Input: part model. Units: mm. Frame: model coordinates. Face numbers are marked on the shaded views. A direction names the side the tool comes from. Coordinates: 2 decimals unless noted, no trailing zeros. Order: outer loops, then holes, each group sorted by start corner. A loop starts at its lowest first (then second) coordinate and runs counter-clockwise, first axis right, second up. Notation, with made-up numbers: (-31, -15) -> (14, -15) arc R23 cw to (14, 21) -> close; hole circle Ø8 at (23.5, -22). An arc over 180 degrees is marked (long way). Use one line per item in the form item = value. Start each with the question number.
1) Section query C-C on y = 15. Output: boundary loops of the cut face in (x, z) (3 decimals).
2) Draft query along X for the marked faces 1, 2, 3 and 4. Return one class per face: pulls with the +X half, pulls with the -X half, needs draft (parallel to the pull), parting line crosses it, or undercut.
3) Section query D-D on y = -16. Output: boundary loops of the cut face in (x, z).
4) Pin query (flat end, axial travel): pin 1 (6 mm diameter, centred on y = -22, z = -9, fed in from -X); pin 2 (9 mm diameter, centred on x = 76.5, z = -70, fed in from +Y); pin 3 (0.9 mm diameter, centred on x = -32.5, y = -1.5, fed in from +Z); pin 4 (25 mm diameter, centred on x = 85.5, y = -15.5, fed in from +Z). Return the tip coordinate at first contact, or that it passes through.
5) Ray query, line 1 along Z through (x, y) = (76.5, 12.75) (3 decimals); line 2 along Z through (x, y) = (76.5, -0.75) (3 decimals); line 3 along Y through (x, z) = (-15, -1.5). Return the intervals inside material, ascending.
6) Access query for the marked faces 5, 6, 7 and 8. Directions: +Z, -Z, +X, -X, +Y, -Y. A direction counts if a zero-diameter tool reaches every point of the face in a straight line with its end or side. Return the directions, or none.
from build123d import *

# Parameters (mm, degrees)
F1_DEPTH       = 25
F2_DEPTH       = 10
F3_DEPTH       = 30
F4_DEPTH       = 20
F5_DEPTH       = 8
F6_SIZE2       = 5
F6_SIZE        = 5
F8_D           = 14.75
F8_CBORE_D     = 22.25
F8_CBORE_DEPTH = 14
F9_R           = 7.49999


# Not quite as in the source:
# - a fillet or chamfer is up to 0.001 mm smaller than in the source, because OpenCascade refuses the exact size


with BuildPart() as f1:
    # F0 (on Front) → F1 (new body)
    with BuildSketch(Plane.XZ):
        with BuildLine():
            Line((106.5, -40), (106.5, 55))
            Line((106.5, 55), (48.7497216032, 55))
            ThreePointArc((48.7497216032, 55), (42.4942891815, 52.8018949761), (38.9888762464, 47.1739130435))
            ThreePointArc((38.9888762464, 47.1739130435), (10.7462120246, -4.2462120246), (-40.6739130435, -32.4888762464))
            ThreePointArc((-40.6739130435, -32.4888762464), (-46.3018949761, -35.9942891815), (-48.5, -42.2497216032))
            Line((-48.5, -42.2497216032), (-48.5, -100))
            Line((-48.5, -100), (46.5, -100))
            Line((46.5, -100), (46.5, -55))
            ThreePointArc((46.5, -55), (50.8933982822, -44.3933982822), (61.5, -40))
            Line((61.5, -40), (106.5, -40))
        make_face()
        with BuildLine():
            ThreePointArc((-29.5, -91), (-36.5710678119, -88.0710678119), (-39.5, -81))
            Line((-39.5, -81), (-39.5, -49.2476414861))
            ThreePointArc((-39.5, -49.2476414861), (-37.481834214, -43.2234965193), (-32.2419354839, -39.630896205))
            ThreePointArc((-32.2419354839, -39.630896205), (17.1101730553, -10.6101730553), (46.130896205, 38.7419354839))
            ThreePointArc((46.130896205, 38.7419354839), (49.7234965193, 43.981834214), (55.7476414861, 46))
            Line((55.7476414861, 46), (87.5, 46))
            ThreePointArc((87.5, 46), (94.5710678119, 43.0710678119), (97.5, 36))
            Line((97.5, 36), (97.5, -21))
            ThreePointArc((97.5, -21), (94.5710678119, -28.0710678119), (87.5, -31))
            Line((87.5, -31), (61.5, -31))
            ThreePointArc((61.5, -31), (44.5294372515, -38.0294372515), (37.5, -55))
            Line((37.5, -55), (37.5, -81))
            ThreePointArc((37.5, -81), (34.5710678119, -88.0710678119), (27.5, -91))
            Line((27.5, -91), (-29.5, -91))
        make_face(mode=Mode.SUBTRACT)
        with BuildLine():
            Line((96.5, 100), (-96.5, 100))
            ThreePointArc((-96.5, 100), (-103.5710678119, 97.0710678119), (-106.5, 90))
            Line((-106.5, 90), (-106.5, -90))
            ThreePointArc((-106.5, -90), (-103.5710678119, -97.0710678119), (-96.5, -100))
            Line((-96.5, -100), (-63.5, -100))
            Line((-63.5, -100), (-63.5, -42.2497216032))
            ThreePointArc((-63.5, -42.2497216032), (-58.0047374401, -26.6111405489), (-43.9347826087, -17.8476082112))
            ThreePointArc((-43.9347826087, -17.8476082112), (0.1396103068, 6.3603896932), (24.3476082112, 50.4347826087))
            ThreePointArc((24.3476082112, 50.4347826087), (33.1111405489, 64.5047374401), (48.7497216032, 70))
            Line((48.7497216032, 70), (106.5, 70))
            Line((106.5, 70), (106.5, 90))
            ThreePointArc((106.5, 90), (103.5710678119, 97.0710678119), (96.5, 100))
        make_face()
        with BuildLine():
            ThreePointArc((14.7304288624, 91), (-11.3221396288, 8.044605666), (-97.5, -3.5187051029))
            Line((-97.5, -3.5187051029), (-97.5, 91))
            Line((-97.5, 91), (14.7304288624, 91))
        make_face(mode=Mode.SUBTRACT)
        with BuildLine():
            Line((-97.5, 91), (-97.5, -3.5187051029))
            ThreePointArc((-97.5, -3.5187051029), (-11.3221396288, 8.044605666), (14.7304288624, 91))
            Line((14.7304288624, 91), (-97.5, 91))
        make_face()
        with BuildLine():
            Line((-39.5, -49.2476414861), (-39.5, -81))
            ThreePointArc((-39.5, -81), (-36.5710678119, -88.0710678119), (-29.5, -91))
            Line((-29.5, -91), (27.5, -91))
            ThreePointArc((27.5, -91), (34.5710678119, -88.0710678119), (37.5, -81))
            Line((37.5, -81), (37.5, -55))
            ThreePointArc((37.5, -55), (44.5294372515, -38.0294372515), (61.5, -31))
            Line((61.5, -31), (87.5, -31))
            ThreePointArc((87.5, -31), (94.5710678119, -28.0710678119), (97.5, -21))
            Line((97.5, -21), (97.5, 36))
            ThreePointArc((97.5, 36), (94.5710678119, 43.0710678119), (87.5, 46))
            Line((87.5, 46), (55.7476414861, 46))
            ThreePointArc((55.7476414861, 46), (49.7234965193, 43.981834214), (46.130896205, 38.7419354839))
            ThreePointArc((46.130896205, 38.7419354839), (17.1101730553, -10.6101730553), (-32.2419354839, -39.630896205))
            ThreePointArc((-32.2419354839, -39.630896205), (-37.481834214, -43.2234965193), (-39.5, -49.2476414861))
        make_face()
        with BuildLine():
            Line((106.5, 55), (106.5, 70))
            Line((106.5, 70), (48.7497216032, 70))
            ThreePointArc((48.7497216032, 70), (33.1111405489, 64.5047374401), (24.3476082112, 50.4347826087))
            ThreePointArc((24.3476082112, 50.4347826087), (0.1396103068, 6.3603896932), (-43.9347826087, -17.8476082112))
            ThreePointArc((-43.9347826087, -17.8476082112), (-58.0047374401, -26.6111405489), (-63.5, -42.2497216032))
            Line((-63.5, -42.2497216032), (-63.5, -100))
            Line((-63.5, -100), (-48.5, -100))
            Line((-48.5, -100), (-48.5, -42.2497216032))
            ThreePointArc((-48.5, -42.2497216032), (-46.3018949761, -35.9942891815), (-40.6739130435, -32.4888762464))
            ThreePointArc((-40.6739130435, -32.4888762464), (10.7462120246, -4.2462120246), (38.9888762464, 47.1739130435))
            ThreePointArc((38.9888762464, 47.1739130435), (42.4942891815, 52.8018949761), (48.7497216032, 55))
            Line((48.7497216032, 55), (106.5, 55))
        make_face()
        with BuildLine():
            Line((106.5, -90), (106.5, -40))
            Line((106.5, -40), (61.5, -40))
            ThreePointArc((61.5, -40), (50.8933982822, -44.3933982822), (46.5, -55))
            Line((46.5, -55), (46.5, -100))
            Line((46.5, -100), (96.5, -100))
            ThreePointArc((96.5, -100), (103.5710678119, -97.0710678119), (106.5, -90))
        make_face()
    extrude(amount=-F1_DEPTH)

    # F0 (on Front) → F2 (join)
    with BuildSketch(Plane.XZ):
        with BuildLine():
            Line((106.5, -90), (106.5, -40))
            Line((106.5, -40), (61.5, -40))
            ThreePointArc((61.5, -40), (50.8933982822, -44.3933982822), (46.5, -55))
            Line((46.5, -55), (46.5, -100))
            Line((46.5, -100), (96.5, -100))
            ThreePointArc((96.5, -100), (103.5710678119, -97.0710678119), (106.5, -90))
        make_face()
    extrude(amount=F2_DEPTH)

    # F0 (on Front) → F3 (join)
    with BuildSketch(Plane.XZ):
        with BuildLine():
            Line((106.5, 55), (106.5, 70))
            Line((106.5, 70), (48.7497216032, 70))
            ThreePointArc((48.7497216032, 70), (33.1111405489, 64.5047374401), (24.3476082112, 50.4347826087))
            ThreePointArc((24.3476082112, 50.4347826087), (0.1396103068, 6.3603896932), (-43.9347826087, -17.8476082112))
            ThreePointArc((-43.9347826087, -17.8476082112), (-58.0047374401, -26.6111405489), (-63.5, -42.2497216032))
            Line((-63.5, -42.2497216032), (-63.5, -100))
            Line((-63.5, -100), (-48.5, -100))
            Line((-48.5, -100), (-48.5, -42.2497216032))
            ThreePointArc((-48.5, -42.2497216032), (-46.3018949761, -35.9942891815), (-40.6739130435, -32.4888762464))
            ThreePointArc((-40.6739130435, -32.4888762464), (10.7462120246, -4.2462120246), (38.9888762464, 47.1739130435))
            ThreePointArc((38.9888762464, 47.1739130435), (42.4942891815, 52.8018949761), (48.7497216032, 55))
            Line((48.7497216032, 55), (106.5, 55))
        make_face()
    extrude(amount=F3_DEPTH)

    # F0 (on Front) → F4 (cut)
    with BuildSketch(Plane.XZ):
        with BuildLine():
            Line((-39.5, -49.2476414861), (-39.5, -81))
            ThreePointArc((-39.5, -81), (-36.5710678119, -88.0710678119), (-29.5, -91))
            Line((-29.5, -91), (27.5, -91))
            ThreePointArc((27.5, -91), (34.5710678119, -88.0710678119), (37.5, -81))
            Line((37.5, -81), (37.5, -55))
            ThreePointArc((37.5, -55), (44.5294372515, -38.0294372515), (61.5, -31))
            Line((61.5, -31), (87.5, -31))
            ThreePointArc((87.5, -31), (94.5710678119, -28.0710678119), (97.5, -21))
            Line((97.5, -21), (97.5, 36))
            ThreePointArc((97.5, 36), (94.5710678119, 43.0710678119), (87.5, 46))
            Line((87.5, 46), (55.7476414861, 46))
            ThreePointArc((55.7476414861, 46), (49.7234965193, 43.981834214), (46.130896205, 38.7419354839))
            ThreePointArc((46.130896205, 38.7419354839), (17.1101730553, -10.6101730553), (-32.2419354839, -39.630896205))
            ThreePointArc((-32.2419354839, -39.630896205), (-37.481834214, -43.2234965193), (-39.5, -49.2476414861))
        make_face()
    extrude(amount=-F4_DEPTH, mode=Mode.SUBTRACT)

    # F0 (on Front) → F5 (join)
    with BuildSketch(Plane.XZ):
        with BuildLine():
            Line((-97.5, 91), (-97.5, -3.5187051029))
            ThreePointArc((-97.5, -3.5187051029), (-11.3221396288, 8.044605666), (14.7304288624, 91))
            Line((14.7304288624, 91), (-97.5, 91))
        make_face()
    extrude(amount=F5_DEPTH)

    # F6
    f6_edges = [f1.edges().sort_by_distance(p)[0] for p in [
        (-41.384786, -8, 91),
        (-97.5, -8, 43.740647),
        (-11.32214, -8, 8.044606),
    ]]
    chamfer(f6_edges, length=F6_SIZE, length2=F6_SIZE2)

    # F8 (through all)
    with Locations(Plane.XZ.offset(10)):
        with Locations((76.5, -70)):
            CounterBoreHole(F8_D / 2, F8_CBORE_D / 2, F8_CBORE_DEPTH)

    # F9 (radius 7.5 in the source; OpenCascade refuses exactly that, so slightly less here)
    f9_edges = [f1.edges().sort_by_distance(p)[0] for p in [
        (-48.5, -30, -71.124861),
        (-63.5, -30, -71.124861),
    ]]
    fillet(f9_edges, radius=F9_R)


solid = f1.part
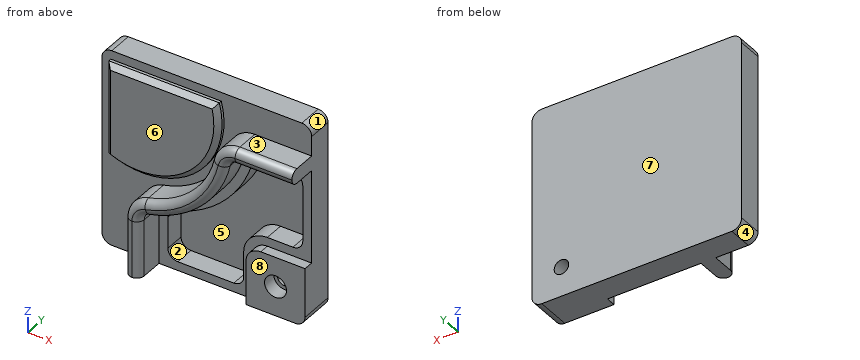
Answers below:
q1.outline = (-106.5, -90) arc R10 ccw to (-96.5, -100) -> (96.5, -100) arc R10 ccw to (106.5, -90) -> (106.5, 90) arc R10 ccw to (96.5, 100) -> (-96.5, 100) arc R10 ccw to (-106.5, 90) -> close; hole (-39.5, -81) arc R10 ccw to (-29.5, -91) -> (27.5, -91) arc R10 ccw to (37.5, -81) -> (37.5, -55) arc R24 cw to (61.5, -31) -> (87.5, -31) arc R10 ccw to (97.5, -21) -> (97.5, 36) arc R10 ccw to (87.5, 46) -> (55.748, 46) arc R10 ccw to (46.131, 38.742) arc R114 cw to (-32.242, -39.631) arc R10 ccw to (-39.5, -49.248) -> close; hole circle Ø14.75 at (76.5, -70)
q2.face_1 = pulls with the +X half
q2.face_2 = undercut
q2.face_3 = needs draft
q2.face_4 = pulls with the -X half
q3.outline = (-63.5, -100) -> (-48.5, -100) -> (-48.5, -42.25) arc R10 cw to (-40.67, -32.49) arc R105 ccw to (38.99, 47.17) arc R10 cw to (48.75, 55) -> (106.5, 55) -> (106.5, 70) -> (48.75, 70) arc R25 ccw to (24.35, 50.43) arc R90 cw to (-43.93, -17.85) arc R25 ccw to (-63.5, -42.25) -> close
q4.pin_1 = -26.41
q4.pin_2 = through
q4.pin_3 = 91
q4.pin_4 = 70
q5.line_1 = -100 to -77.375, -62.625 to -31, 46 to 100
q5.line_2 = -100 to -81.125, -58.875 to -40, 55 to 70
q5.line_3 = 0 to 25
q6.face_5 = -Y
q6.face_6 = +Z, -X, -Y
q6.face_7 = +Z, -Z, +X, -X, +Y
q6.face_8 = -Z, +X, -Y
